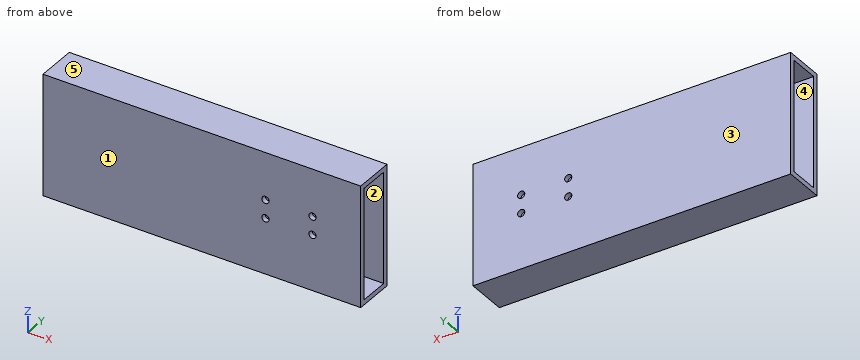
```python
from build123d import *

# Parameters (mm, degrees)
SKETCH1_W            = 152.4
SKETCH1_H            = 50.8
SKETCH1_W_2          = 139.7
SKETCH1_H_2          = 38.1
BOSS_EXTRUDE1_DEPTH  = 400
M8_CLEARANCE_HOLE1_D = 9


with BuildPart() as part:
    # Sketch1 → Boss-Extrude1 (new body)
    with BuildSketch(Plane(origin=(0, 0, 0), x_dir=(0, 0, -1), z_dir=(1, 0, 0))):
        Rectangle(SKETCH1_W, SKETCH1_H)
        Rectangle(SKETCH1_W_2, SKETCH1_H_2, mode=Mode.SUBTRACT)
    extrude(amount=BOSS_EXTRUDE1_DEPTH)

    # M8 Clearance Hole1 (through all)
    with Locations(Plane(origin=(0, -25.4, 0), x_dir=(-1, 0, 0), z_dir=(0, -1, 0))):
        with Locations((-280.09, -16.73), (-280.09, 6.27), (-339.29, 6.27), (-339.29, -16.73)):
            Hole(M8_CLEARANCE_HOLE1_D / 2)


solid = part.part
```
The listing builds one solid part. Answer for the finished solid, in the listing's coordinates (mm). Face numbers are marked on the shaded views. A direction names the side the tool comes from. Give positions to 0.01 mm unless a question says otherwise; leave off trailing zeros. Write each loop counter-clockwise with the first axis right and the second up, starting at its lowest first coordinate (ties: lowest second). Pieces come first, ordered by that corner, then holes. Notation, with made-up numbers: (74, 89) -> (115, 89) arc R10 ccw to (115, 104) -> close; hole circle Ø5 at (53, 46.5). An arc over 180 degrees is marked (long way). Write item = value, one per line. Start each with the question number.
1) Which of the six approach directions +Z, -Z, +X, -X, +Y, -Y give full straight-line access (tool end or side, diameter ignored) to the marked faces 1 and 2?
2) The part is cut by section D-D, the plane z = 16.73. Determine the outline of the cut face in (x, y), and give its area (3 significant figures).
3) The part is cut by section C-C, the plane y = 3.5. Determine the outline of the cut face in (x, z), and give its area (3 significant figures).
4) The part is cut by section A-A, the plane z = -31. Determine the outline of the cut face in (x, y).
5) Determine the mould class of the marked faces 3, 4 and 5 for opening direction Y: +Y half, -Y half, draft (parallel to the pull), parting line (faces both ways), or undercut.
6) Straight lines are drawn through the part: line 1 along Z through (x, y) = (280.09, -23.25); line 2 along X through (y, z) = (24, 16.73); line 3 along Y through (x, z) = (172, 47.5). For each, find the intervals that lie inside material, in ascending order.
7) The part is cut by section B-B, the plane x = 88. Determine the outline of the cut face in (y, z), and give its area (3 significant figures).
Solutions:
q1.face_1 = +Z, -Z, +X, -X, -Y
q1.face_2 = +X, -X
q2.outline = (0, -25.4) -> (275.59, -25.4) -> (275.59, -19.05) -> (0, -19.05) -> close; (0, 19.05) -> (275.59, 19.05) -> (275.59, 25.4) -> (0, 25.4) -> close; (284.59, -25.4) -> (334.79, -25.4) -> (334.79, -19.05) -> (284.59, -19.05) -> close; (284.59, 19.05) -> (334.79, 19.05) -> (334.79, 25.4) -> (284.59, 25.4) -> close; (343.79, -25.4) -> (400, -25.4) -> (400, -19.05) -> (343.79, -19.05) -> close; (343.79, 19.05) -> (400, 19.05) -> (400, 25.4) -> (343.79, 25.4) -> close
q2.area = 4,850 mm²
q3.outline = (0, -76.2) -> (400, -76.2) -> (400, -69.85) -> (0, -69.85) -> close; (0, 69.85) -> (400, 69.85) -> (400, 76.2) -> (0, 76.2) -> close
q3.area = 5,080 mm²
q4.outline = (0, -25.4) -> (400, -25.4) -> (400, -19.05) -> (0, -19.05) -> close; (0, 19.05) -> (400, 19.05) -> (400, 25.4) -> (0, 25.4) -> close
q5.face_3 = +Y half
q5.face_4 = undercut
q5.face_5 = draft
q6.line_1 = -76.2 to -10.77, -1.77 to 12.23, 21.23 to 76.2
q6.line_2 = 0 to 275.59, 284.59 to 334.79, 343.79 to 400
q6.line_3 = -25.4 to -19.05, 19.05 to 25.4
q7.outline = (-25.4, -76.2) -> (25.4, -76.2) -> (25.4, 76.2) -> (-25.4, 76.2) -> close; hole (-19.05, -69.85) -> (19.05, -69.85) -> (19.05, 69.85) -> (-19.05, 69.85) -> close
q7.area = 2,420 mm²
